Source: CAD feature listing. Evaluate the final solid. Frame: model axes, mm. Face numbers are marked on the shaded views. A direction names the side the tool comes from. Give positions to 0.01 mm unless a question says otherwise; leave off trailing zeros. Order: outer loops, then holes, each group sorted by start corner. A loop starts at its lowest first (then second) coordinate and runs counter-clockwise, first axis right, second up.
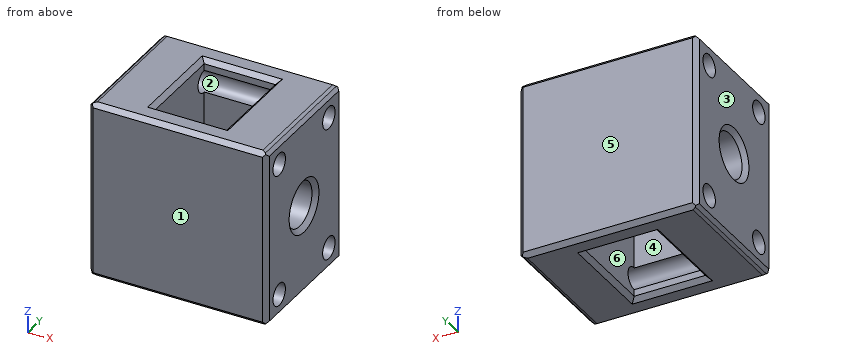
from build123d import *

# Parameters (mm, degrees)
F0_W         = 150
F0_H         = 200
F0_R         = 25
F1_DEPTH     = 200
F2_SIZE      = 5
F3_R         = 12.5
F4_DEPTH     = 200.001
F5_W         = 80
F5_H         = 100
F6_DEPTH     = 200.001
F7_T1_DEPTH  = 215.7168298797
F7_T3_DEPTH  = 161.2857086021
F7_T5_DEPTH  = 100
F7_T7_DEPTH  = 80
F7_T13_DEPTH = 112.8584149398
F7_T17_DEPTH = 92.8584149398
F7_T24_DEPTH = 112.8584149398
F7_T28_DEPTH = 92.8584149398
F7_T35_DEPTH = 92.8584149398
F7_T39_DEPTH = 112.8584149398
F7_T46_DEPTH = 112.8584149398
F7_T50_DEPTH = 92.8584149398
F7_T57_DEPTH = 112.8584149398
F7_T61_DEPTH = 92.8584149398
F7_T68_DEPTH = 112.8584149398
F7_T72_DEPTH = 92.8584149398
F7_T79_DEPTH = 112.8584149398
F7_T83_DEPTH = 92.8584149398
F7_T90_DEPTH = 112.8584149398
F7_T94_DEPTH = 92.8584149398


# Not quite as in the source:
# - a fillet or chamfer that OpenCascade refuses, or shapes differently, is made with other operations: its cross-section is extruded or revolved along the edge and cut away or added


with BuildPart() as f1:
    # F0 (on Right) → F1 (new body)
    with BuildSketch(Plane.YZ):
        Rectangle(F0_W, F0_H)
        Circle(F0_R, mode=Mode.SUBTRACT)
    extrude(amount=-F1_DEPTH)

    # F2
    f2_edges = [f1.edges().sort_by_distance(p)[0] for p in [
        (0, 0, -100),
        (0, 75, 0),
        (0, 0, 100),
        (0, -75, 0),
        (0, -25, 0),
        (-200, 0, -100),
        (-200, 75, 0),
        (-200, 0, 100),
        (-200, -75, 0),
        (-200, -25, 0),
    ]]
    chamfer(f2_edges, length=F2_SIZE)

    # F3 (on face) → F4 (cut, through all)
    with BuildSketch(Plane(origin=(-200, 0, 0), x_dir=(0, -1, 0), z_dir=(-1, 0, 0))):
        with Locations((-50, -75)):
            Circle(F3_R)
        with Locations((-50, 75)):
            Circle(F3_R)
        with Locations((50, -75)):
            Circle(F3_R)
        with Locations((50, 75)):
            Circle(F3_R)
    extrude(amount=-F4_DEPTH, mode=Mode.SUBTRACT)

    # F5 (on face) → F6 (cut, through all)
    with BuildSketch(Plane(origin=(0, 0, -100), x_dir=(1, 0, 0), z_dir=(0, 0, -1))):
        with Locations((-100, 0)):
            Rectangle(F5_W, F5_H)
    extrude(amount=-F6_DEPTH, mode=Mode.SUBTRACT)

    # F7: chamfer of 5 on 16 edges, made by hand

    # F7_s2 → F7_t1 (cut)
    with BuildSketch(Plane.YZ.offset(-207.8584149398)):
        Polygon((-70, -100), (-75, -95), (-75, -100), align=None)
        Polygon((70, -100), (75, -95), (75, -100), align=None)
        Polygon((75, 95), (70, 100), (75, 100), align=None)
        Polygon((-75, 95), (-70, 100), (-75, 100), align=None)
    extrude(amount=F7_T1_DEPTH, mode=Mode.SUBTRACT)

    # F7_s4 → F7_t3 (cut)
    with BuildSketch(Plane.XZ.offset(-80.6428543011)):
        Polygon((-7.0710678119, -100), (-3.5355339059, -98.5355339059), (-5, -100), align=None)
        Polygon((-192.9289321881, -100), (-196.4644660941, -98.5355339059), (-195, -100), align=None)
        Polygon((-7.0710678119, 100), (-3.5355339059, 98.5355339059), (-5, 100), align=None)
        Polygon((-192.9289321881, 100), (-196.4644660941, 98.5355339059), (-195, 100), align=None)
    extrude(amount=F7_T3_DEPTH, mode=Mode.SUBTRACT)

    # F7_s6 → F7_t5 (cut)
    with BuildSketch(Plane.XZ.offset(-50)):
        Polygon((-55, -100), (-60, -95), (-60, -100), align=None)
        Polygon((-145, -100), (-140, -95), (-140, -100), align=None)
        Polygon((-60, 95), (-55, 100), (-60, 100), align=None)
        Polygon((-140, 95), (-145, 100), (-140, 100), align=None)
    extrude(amount=F7_T5_DEPTH, mode=Mode.SUBTRACT)

    # F7_s8 → F7_t7 (cut)
    with BuildSketch(Plane.YZ.offset(-140)):
        Polygon((-55, -100), (-50, -95), (-50, -100), align=None)
        Polygon((55, -100), (50, -95), (50, -100), align=None)
        Polygon((55, 100), (50, 95), (50, 100), align=None)
        Polygon((-55, 100), (-50, 95), (-50, 100), align=None)
    extrude(amount=F7_T7_DEPTH, mode=Mode.SUBTRACT)


with BuildPart() as f7_tool11:
    # F7_s12 → F7_t13 (new body)
    with BuildSketch(Plane.XZ.offset(-62.8584149398)):
        Polygon((-55, -100), (-60, -95), (-60, -100), align=None)
    extrude(amount=F7_T13_DEPTH)

    split(bisect_by=Plane.XZ.offset(-50), keep=Keep.BOTTOM)


with BuildPart() as f7_tool15:
    # F7_s16 → F7_t17 (new body)
    with BuildSketch(Plane.YZ.offset(-140)):
        Polygon((55, -100), (50, -95), (50, -100), align=None)
    extrude(amount=F7_T17_DEPTH)

    split(bisect_by=Plane.YZ.offset(-60), keep=Keep.TOP)


with BuildPart() as f7_tool11_1:
    add(f7_tool11.part)

    # F7_t19: intersect F7_tool15
    add(f7_tool15.part, mode=Mode.INTERSECT)


with BuildPart() as f1_1:
    add(f1.part)

    # F7_t9: cut F7_tool11
    add(f7_tool11_1.part, mode=Mode.SUBTRACT)


with BuildPart() as f7_tool22:
    # F7_s23 → F7_t24 (new body)
    with BuildSketch(Plane.XZ.offset(-50)):
        Polygon((-55, -100), (-60, -95), (-60, -100), align=None)
    extrude(amount=F7_T24_DEPTH)

    split(bisect_by=Plane.XZ.offset(50), keep=Keep.TOP)


with BuildPart() as f7_tool26:
    # F7_s27 → F7_t28 (new body)
    with BuildSketch(Plane.YZ.offset(-47.1415850602)):
        Polygon((-55, -100), (-50, -95), (-50, -100), align=None)
    extrude(amount=-F7_T28_DEPTH)

    split(bisect_by=Plane.YZ.offset(-60), keep=Keep.TOP)


with BuildPart() as f7_tool22_1:
    add(f7_tool22.part)

    # F7_t30: intersect F7_tool26
    add(f7_tool26.part, mode=Mode.INTERSECT)


with BuildPart() as f1_2:
    add(f1_1.part)

    # F7_t20: cut F7_tool22
    add(f7_tool22_1.part, mode=Mode.SUBTRACT)


with BuildPart() as f7_tool33:
    # F7_s34 → F7_t35 (new body)
    with BuildSketch(Plane.YZ.offset(-60)):
        Polygon((-55, -100), (-50, -95), (-50, -100), align=None)
    extrude(amount=-F7_T35_DEPTH)

    split(bisect_by=Plane.YZ.offset(-140), keep=Keep.BOTTOM)


with BuildPart() as f7_tool37:
    # F7_s38 → F7_t39 (new body)
    with BuildSketch(Plane.XZ.offset(62.8584149398)):
        Polygon((-145, -100), (-140, -95), (-140, -100), align=None)
    extrude(amount=-F7_T39_DEPTH)

    split(bisect_by=Plane.XZ.offset(50), keep=Keep.TOP)


with BuildPart() as f7_tool33_1:
    add(f7_tool33.part)

    # F7_t41: intersect F7_tool37
    add(f7_tool37.part, mode=Mode.INTERSECT)


with BuildPart() as f1_3:
    add(f1_2.part)

    # F7_t31: cut F7_tool33
    add(f7_tool33_1.part, mode=Mode.SUBTRACT)


with BuildPart() as f7_tool44:
    # F7_s45 → F7_t46 (new body)
    with BuildSketch(Plane.XZ.offset(50)):
        Polygon((-145, -100), (-140, -95), (-140, -100), align=None)
    extrude(amount=-F7_T46_DEPTH)

    split(bisect_by=Plane.XZ.offset(-50), keep=Keep.BOTTOM)


with BuildPart() as f7_tool48:
    # F7_s49 → F7_t50 (new body)
    with BuildSketch(Plane.YZ.offset(-152.8584149398)):
        Polygon((55, -100), (50, -95), (50, -100), align=None)
    extrude(amount=F7_T50_DEPTH)

    split(bisect_by=Plane.YZ.offset(-140), keep=Keep.BOTTOM)


with BuildPart() as f7_tool44_1:
    add(f7_tool44.part)

    # F7_t52: intersect F7_tool48
    add(f7_tool48.part, mode=Mode.INTERSECT)


with BuildPart() as f1_4:
    add(f1_3.part)

    # F7_t42: cut F7_tool44
    add(f7_tool44_1.part, mode=Mode.SUBTRACT)


with BuildPart() as f7_tool55:
    # F7_s56 → F7_t57 (new body)
    with BuildSketch(Plane.XZ.offset(62.8584149398)):
        Polygon((-60, 95), (-55, 100), (-60, 100), align=None)
    extrude(amount=-F7_T57_DEPTH)

    split(bisect_by=Plane.XZ.offset(50), keep=Keep.TOP)


with BuildPart() as f7_tool59:
    # F7_s60 → F7_t61 (new body)
    with BuildSketch(Plane.YZ.offset(-140)):
        Polygon((-55, 100), (-50, 95), (-50, 100), align=None)
    extrude(amount=F7_T61_DEPTH)

    split(bisect_by=Plane.YZ.offset(-60), keep=Keep.TOP)


with BuildPart() as f7_tool55_1:
    add(f7_tool55.part)

    # F7_t63: intersect F7_tool59
    add(f7_tool59.part, mode=Mode.INTERSECT)


with BuildPart() as f1_5:
    add(f1_4.part)

    # F7_t53: cut F7_tool55
    add(f7_tool55_1.part, mode=Mode.SUBTRACT)


with BuildPart() as f7_tool66:
    # F7_s67 → F7_t68 (new body)
    with BuildSketch(Plane.XZ.offset(50)):
        Polygon((-60, 95), (-55, 100), (-60, 100), align=None)
    extrude(amount=-F7_T68_DEPTH)

    split(bisect_by=Plane.XZ.offset(-50), keep=Keep.BOTTOM)


with BuildPart() as f7_tool70:
    # F7_s71 → F7_t72 (new body)
    with BuildSketch(Plane.YZ.offset(-47.1415850602)):
        Polygon((55, 100), (50, 95), (50, 100), align=None)
    extrude(amount=-F7_T72_DEPTH)

    split(bisect_by=Plane.YZ.offset(-60), keep=Keep.TOP)


with BuildPart() as f7_tool66_1:
    add(f7_tool66.part)

    # F7_t74: intersect F7_tool70
    add(f7_tool70.part, mode=Mode.INTERSECT)


with BuildPart() as f1_6:
    add(f1_5.part)

    # F7_t64: cut F7_tool66
    add(f7_tool66_1.part, mode=Mode.SUBTRACT)


with BuildPart() as f7_tool77:
    # F7_s78 → F7_t79 (new body)
    with BuildSketch(Plane.XZ.offset(-62.8584149398)):
        Polygon((-140, 95), (-145, 100), (-140, 100), align=None)
    extrude(amount=F7_T79_DEPTH)

    split(bisect_by=Plane.XZ.offset(-50), keep=Keep.BOTTOM)


with BuildPart() as f7_tool81:
    # F7_s82 → F7_t83 (new body)
    with BuildSketch(Plane.YZ.offset(-60)):
        Polygon((55, 100), (50, 95), (50, 100), align=None)
    extrude(amount=-F7_T83_DEPTH)

    split(bisect_by=Plane.YZ.offset(-140), keep=Keep.BOTTOM)


with BuildPart() as f7_tool77_1:
    add(f7_tool77.part)

    # F7_t85: intersect F7_tool81
    add(f7_tool81.part, mode=Mode.INTERSECT)


with BuildPart() as f1_7:
    add(f1_6.part)

    # F7_t75: cut F7_tool77
    add(f7_tool77_1.part, mode=Mode.SUBTRACT)


with BuildPart() as f7_tool88:
    # F7_s89 → F7_t90 (new body)
    with BuildSketch(Plane.XZ.offset(-50)):
        Polygon((-140, 95), (-145, 100), (-140, 100), align=None)
    extrude(amount=F7_T90_DEPTH)

    split(bisect_by=Plane.XZ.offset(50), keep=Keep.TOP)


with BuildPart() as f7_tool92:
    # F7_s93 → F7_t94 (new body)
    with BuildSketch(Plane.YZ.offset(-152.8584149398)):
        Polygon((-55, 100), (-50, 95), (-50, 100), align=None)
    extrude(amount=F7_T94_DEPTH)

    split(bisect_by=Plane.YZ.offset(-140), keep=Keep.BOTTOM)


with BuildPart() as f7_tool88_1:
    add(f7_tool88.part)

    # F7_t96: intersect F7_tool92
    add(f7_tool92.part, mode=Mode.INTERSECT)


with BuildPart() as f1_8:
    add(f1_7.part)

    # F7_t86: cut F7_tool88
    add(f7_tool88_1.part, mode=Mode.SUBTRACT)


solid = f1_8.part
1) Reachability of the marked faces 5 and 6 from +Z, -Z, +X, -X, +Y, -Y: full face, straight path, thin tool, end or side. Return the list, or none.
Checks:
face 5: +Z, -Z, +X, -X, +Y
face 6: +Z, -Z
2) Section query B-B on z = 75. Output: boundary loops of the cut face in (x, y).
Checks:
outline: (-200, -70) - (-195, -75) - (-5, -75) - (0, -70) - (0, -62.5) - (-200, -62.5) - close; (-200, -37.5) - (-140, -37.5) - (-140, 37.5) - (-200, 37.5) - close; (-200, 62.5) - (0, 62.5) - (0, 70) - (-5, 75) - (-195, 75) - (-200, 70) - close; (-60, -37.5) - (0, -37.5) - (0, 37.5) - (-60, 37.5) - close
3) Section query D-D on z = 0. Output: boundary loops of the cut face in (x, y).
Checks:
outline: (-200, -70) - (-195, -75) - (-5, -75) - (0, -70) - (0, -30) - (-5, -25) - (-60, -25) - (-60, -50) - (-140, -50) - (-140, -25) - (-195, -25) - (-200, -30) - close; (-200, 30) - (-195, 25) - (-140, 25) - (-140, 50) - (-60, 50) - (-60, 25) - (-5, 25) - (0, 30) - (0, 70) - (-5, 75) - (-195, 75) - (-200, 70) - close
4) First-contact query: pin 1 Ø3 at (x, y) = (-126.5, -49.5) entering from -Z; pin 2 Ø1 at (y, z) = (21.5, 17) entering from +X. Flat tips, straight axial feed; report the tip coordinate or a pass-through.
Checks:
pin 1: stops at z = -96
pin 2: stops at x = -2.09
5) Ray query, L1, parallel to Z at x = -150, y = 50; L2, parallel to X at y = 9, z = -54.5; L3, parallel to Y at x = -185, z = 74.5. Return the intervals inside material, ascending.
Checks:
L1: z = -100 to -87.5, -62.5 to 62.5, 87.5 to 100
L2: x = -200 to -140, -60 to 0
L3: y = -75 to -62.49, -37.51 to 37.51, 62.49 to 75
6) Pull-direction query (Y, two-part tool) for the marked faces 1, 2, 3 and 4; classes: +Y half, -Y half, draft (parallel to the pull), parting line (faces both ways), or undercut.
Checks:
face 1: -Y half
face 2: undercut
face 3: draft
face 4: undercut
7) Section query C-C on x = -155. Output: boundary loops of the cut face in (y, z), and give its area (3 significant figures).
Checks:
outline: (-75, -95) - (-70, -100) - (70, -100) - (75, -95) - (75, 95) - (70, 100) - (-70, 100) - (-75, 95) - close; hole circle Ø25 at (-50, -75); hole circle Ø25 at (-50, 75); hole circle Ø50 at (0, 0); hole circle Ø25 at (50, -75); hole circle Ø25 at (50, 75)
area: 26,000 mm2
8) Section query A-A on x = -86. Output: boundary loops of the cut face in (y, z), and give its area (3 significant figures).
Checks:
outline: (-75, -95) - (-70, -100) - (-55, -100) - (-50, -95) - (-50, -87.5) arc R12.5 cw to (-50, -62.5) - (-50, 62.5) arc R12.5 cw to (-50, 87.5) - (-50, 95) - (-55, 100) - (-70, 100) - (-75, 95) - close; (50, -95) - (55, -100) - (70, -100) - (75, -95) - (75, 95) - (70, 100) - (55, 100) - (50, 95) - (50, 87.5) arc R12.5 cw to (50, 62.5) - (50, -62.5) arc R12.5 cw to (50, -87.5) - close
area: 8,920 mm2
